Check sheet for the modelled part. Datum: model origin and axes. Units: mm. A direction names the side the tool comes from. Give positions to 0.01 mm unless a question says otherwise; leave off trailing zeros. Order: outer loops, then holes, each group sorted by start corner. A loop starts at its lowest first (then second) coordinate and runs counter-clockwise, first axis right, second up. Notation, with made-up numbers: (24.25, 13.5) -> (69.25, 13.5) arc R9 ccw to (69.25, 29.5) -> close; hole circle Ø3 at (-7, 39). An arc over 180 degrees is marked (long way). One line per question, with ' | ' between items.
```python
from build123d import *

# Parameters (mm, degrees)
SKETCH_R         = 6
PAD_DEPTH        = 3
SKETCH002_R      = 3.25
PAD001_DEPTH     = 3
HOLE_D           = 4.5
HOLE_DEPTH       = 25
HOLE_CBORE_D     = 7
HOLE_CBORE_DEPTH = 2
FILLET_R         = 2


with BuildPart() as part:
    # Sketch → Pad (new body)
    with BuildSketch(Plane.XY):
        Circle(SKETCH_R)
    extrude(amount=PAD_DEPTH)

    # Sketch002 → Pad001 (join)
    with BuildSketch(Plane(origin=(0, 0, 0), x_dir=(1, 0, 0), z_dir=(0, 0, -1))):
        Circle(SKETCH002_R)
    extrude(amount=PAD001_DEPTH)

    # Hole
    with Locations(Plane.XY.offset(3)):
        with Locations((0, 0)):
            CounterBoreHole(HOLE_D / 2, HOLE_CBORE_D / 2, HOLE_CBORE_DEPTH, depth=HOLE_DEPTH)

    # Fillet
    fillet_edges = [part.edges().sort_by_distance(p)[0] for p in [
        (-6, 0, 3),
    ]]
    fillet(fillet_edges, radius=FILLET_R)


solid = part.part
```
Q1. Thickness scan on line 1 (Y direction, x = 0, z = -1.1); line 2 (Z direction, x = 2.5, y = -1.5); line 3 (Y direction, x = 0, z = 0.1). Record the ranges inside material, lowest first.
Result sheet:
line 1: y = -3.25 to -2.25, 2.25 to 3.25 | line 2: z = -3 to 1 | line 3: y = -6 to -2.25, 2.25 to 6
Q2. Section check C-C (z = 0.15). Enter the section's corners in (x, y).
Result sheet:
outline: circle Ø12 at (0, 0); hole circle Ø4.5 at (0, 0)
Q3. Mould release check, pull along Y, two halves, no side actions. Record for faces 1 (the face through (2.3, -0.7, 1)), 2 (the face through (-2.579, 1.978, -1.479)), 3 (the face through (3, -3, 0)): pulls with the +Y half, pulls with the -Y half, needs draft (parallel to the pull), parting line crosses it, or undercut.
Result sheet:
face 1: undercut | face 2: parting line crosses it | face 3: needs draft
Q4. Depth check by flat-ended pin: pin 1 Ø5 at (x, y) = (0, 0) entering from +Z; pin 2 Ø1.5 at (x, z) = (1, -1.5) entering from -Y; pin 3 Ø1.5 at (y, z) = (4.5, -1) entering from +X; pin 4 Ø3 at (x, z) = (-2.5, -0.5) entering from +Y. Enter the tip coordinate at first touch or a pass-through.
Result sheet:
pin 1: stops at z = 1 | pin 2: stops at y = -3.24 | pin 3: passes through | pin 4: stops at y = 5.9
Q5. Section check D-D (z = -1.9). Enter the section's corners in (x, y), and give its area (3 significant figures).
Result sheet:
outline: circle Ø6.5 at (0, 0); hole circle Ø4.5 at (0, 0) | area: 17.3 mm2
Q6. Section check A-A (x = 0). Enter the section's corners in (y, z), and give its area (3 significant figures).
Result sheet:
outline: (-6, 0) -> (-3.25, 0) -> (-3.25, -3) -> (-2.25, -3) -> (-2.25, 1) -> (-3.5, 1) -> (-3.5, 3) -> (-4, 3) arc R2 ccw to (-6, 1) -> close; (2.25, -3) -> (3.25, -3) -> (3.25, 0) -> (6, 0) -> (6, 1) arc R2 ccw to (4, 3) -> (3.5, 3) -> (3.5, 1) -> (2.25, 1) -> close | area: 21.8 mm2
Q7. Access from +Z, -Z, +X, -X, +Y, -Y to the whole of each face (thin tool, end or side, straight path). Record for faces 4 (the face through (3.233, -1.341, 2.014)), 5 (the face through (-5.994, 0.264, 0.493)).
Result sheet:
face 4: +Z | face 5: +Z, -Z
